Verification items for this drawing (mm, ordinates from the low corner). A direction names the side the tool comes from. Give positions to 0.01 mm unless a question says otherwise; leave off trailing zeros. Loops run counter-clockwise (first coordinate to the right, second up) from the corner with the lowest first, then second, coordinate; pieces in that order, holes last. Notation, with made-up numbers: M 44,54.5 L 101,54.5 A13 ccw 101,70.5 Z; hole C -24,-38.75 d1. An arc over 180 degrees is marked long. Answer in a Markdown table with one row per item.
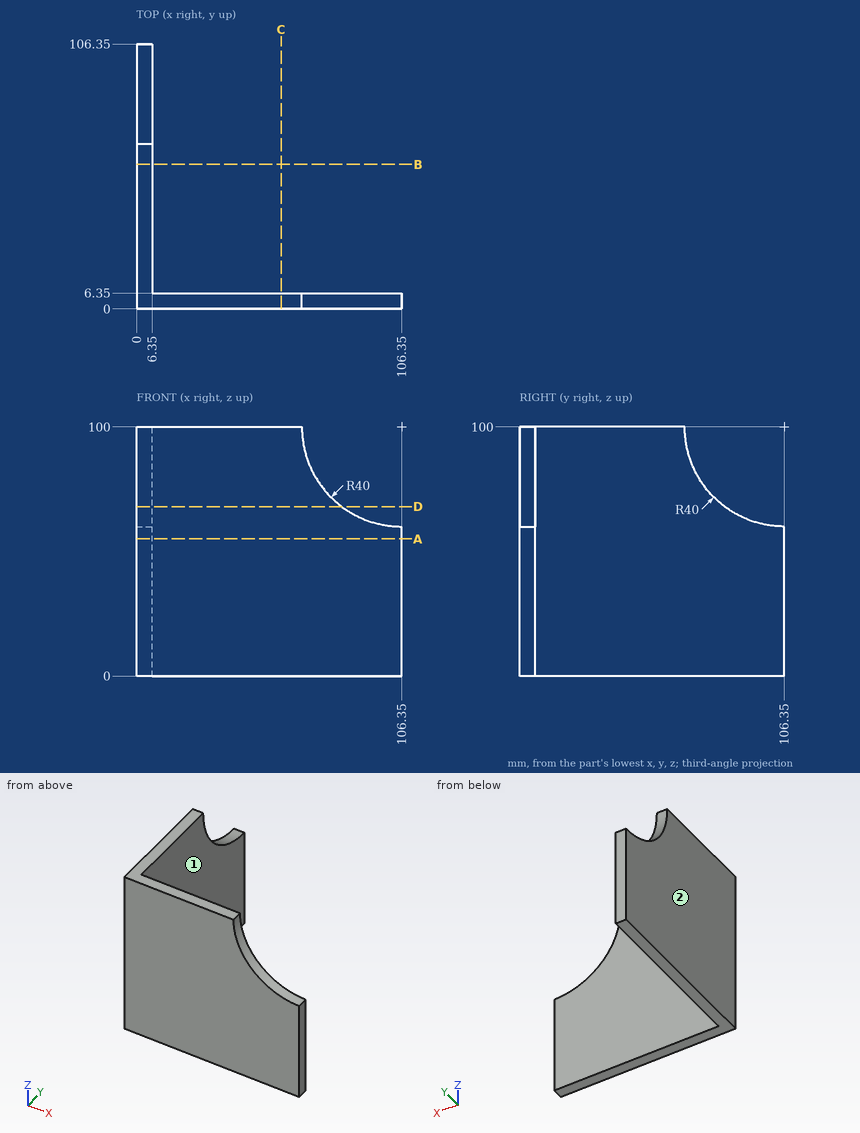
Item 1: Scan lines: L1, parallel to Y at x = 14, z = 50; L2, parallel to Y at x = 6, z = 67. Record each from-to range of solid material in increasing order. Write a range as [from, to].
Reported:
| item | result |
|---|---|
| L1 | y = [0, 6.35] |
| L2 | y = [0, 83.74] |
Item 2: Tool access check on the marked faces 1 and 2. Record the directions out of +Z, -Z, +X, -X, +Y, -Y that give a thin tool (end or side, any length) a straight path to the whole face; none if there is none.
Reported:
| item | result |
|---|---|
| face 1 | +Z, -Z, +X, +Y |
| face 2 | +Z, -Z, -X, +Y, -Y |
Item 3: Sectioned sample at B-B (y = 58). Record the cut outline in (x, z), and give its area (3 significant figures).
Reported:
| item | result |
|---|---|
| outline | M 0,0 L 6.35,0 L 6.35,100 L 0,100 Z |
| area | 635 mm^2 |
Item 4: Sectioned sample at A-A (z = 55). Record the cut outline in (x, y), and give its area (3 significant figures).
Reported:
| item | result |
|---|---|
| outline | M 0,0 L 106.35,0 L 106.35,6.35 L 6.35,6.35 L 6.35,106.35 L 0,106.35 Z |
| area | 1,310 mm^2 |
Item 5: Go/stop test with flat-tipped pins: pin 1 (6 mm diameter, centred on y = 14, z = 17.5, fed in from +X); pin 2 (1.5 mm diameter, centred on x = 58, z = 19, fed in from +Y). Record where each tip stops, or that it passes through.
Reported:
| item | result |
|---|---|
| pin 1 | stops at x = 6.35 |
| pin 2 | stops at y = 6.35 |
Item 6: Sectioned sample at D-D (z = 68). Record the cut outline in (x, y).
Reported:
| item | result |
|---|---|
| outline | M 0,0 L 82.35,0 L 82.35,6.35 L 6.35,6.35 L 6.35,82.35 L 0,82.35 Z |
